Source: CAD feature listing. Evaluate the final solid. Frame: model axes, mm. Round coordinates to 2 decimals unless told otherwise and drop trailing zeros. Order: outer loops, then holes, each group sorted by start corner. A loop starts at its lowest first (then second) coordinate and runs counter-clockwise, first axis right, second up. Notation, with made-up numbers: (39.25, 31) - (53.25, 31) arc R23 ccw to (53.25, 57) - close; hole circle Ø11 at (67.5, -28). An arc over 180 degrees is marked (long way). Put each result on its own line as item: value. Start each with the question number.
1) Section A-A on x = -213.5. Output: boundary loops of the cut face in (y, z), then the cut area to 3 significant figures.
2) Contact query for flat-ended pins moving along their axis: P1, Ø4, axis at x = 238.5, z = -1.5, coming from the -Y side; P2, Ø3, axis at x = 164, z = 42.5, coming from the -Y side; P3, Ø2, axis at x = 232, z = 31, coming from the -Y side. Output: stop coordinate, or through.
3) Line query: probe 1 along Y at (x, z) = (154.5, -5); probe 2 along Y at (x, z) = (-321, 6.5); probe 3 along Z at (x, y) = (-262, 8.5). Output: solid intervals per line, ascending. Write a range as [from, to].
4) Section B-B on z = -45. Output: boundary loops of the cut face in (x, y).
5) Section C-C on y = 2.75. Output: boundary loops of the cut face in (x, z), then the cut area to 4 significant figures.
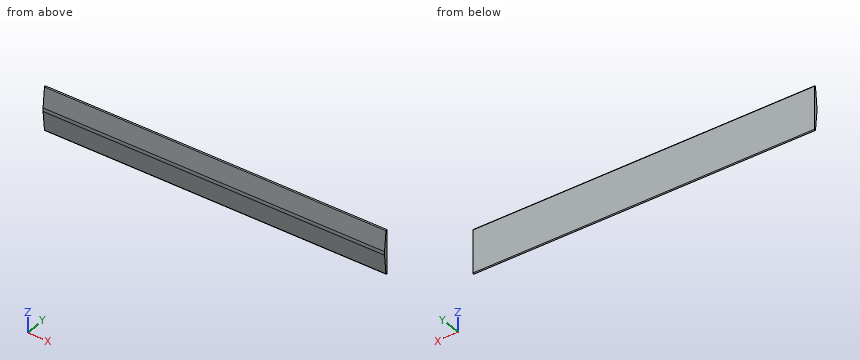
Autodesk Inventor part; units mm, degrees
ref_plane "YZ Plane" through (0, 0, 0) normal (1, 0, 0) x (0, 1, 0)
ref_plane "XZ Plane" through (0, 0, 0) normal (0, 1, 0) x (-1, 0, 0)
ref_plane "XY Plane" through (0, 0, 0) normal (0, 0, 1) x (1, 0, 0)
sketch "スケッチ1" plane through (0, 0, 0) normal (1, 0, 0) x (0, 1, 0)
  line L0 (10, 100) -> (10, -100)
  line L1 (10, -100) -> (0, 0)
  line L2 (0, 0) -> (10, 100)
  line L3 (-2, 0) -> (12, 0)
  point P0 (10, 0)
  dimension "d0" = 200
  dimension "d5" = 10
extrude "押し出し1" add sketch "スケッチ1" along normal mid plane 950
fillet "フィレット1" radius 2 2 edges at (0, 10, 100) (0, 10, -100)
fillet "フィレット1" radius 50 1 edges at (0, 0, 0)
properties part number "foward_flap" material "CFRP"
Answer sheet:
1. outline: (0.5, -4.98) - (6.01, -60.1) arc R2 ccw to (10, -59.9) - (10, 59.9) arc R2 ccw to (6.01, 60.1) - (0.5, 4.98) arc R50 ccw to start
1. area: 851 mm^2
2. P1: y = 0.25
2. P2: y = 4.1
2. P3: y = 3
3. probe 1: [0.5, 10]
3. probe 2: [0.65, 10]
3. probe 3: [-61.84, 61.84]
4. outline: (-475, 4.5) - (475, 4.5) - (475, 10) - (-475, 10) - close
5. outline: (-475, -27.5) - (475, -27.5) - (475, 27.5) - (-475, 27.5) - close
5. area: 52,250 mm^2
